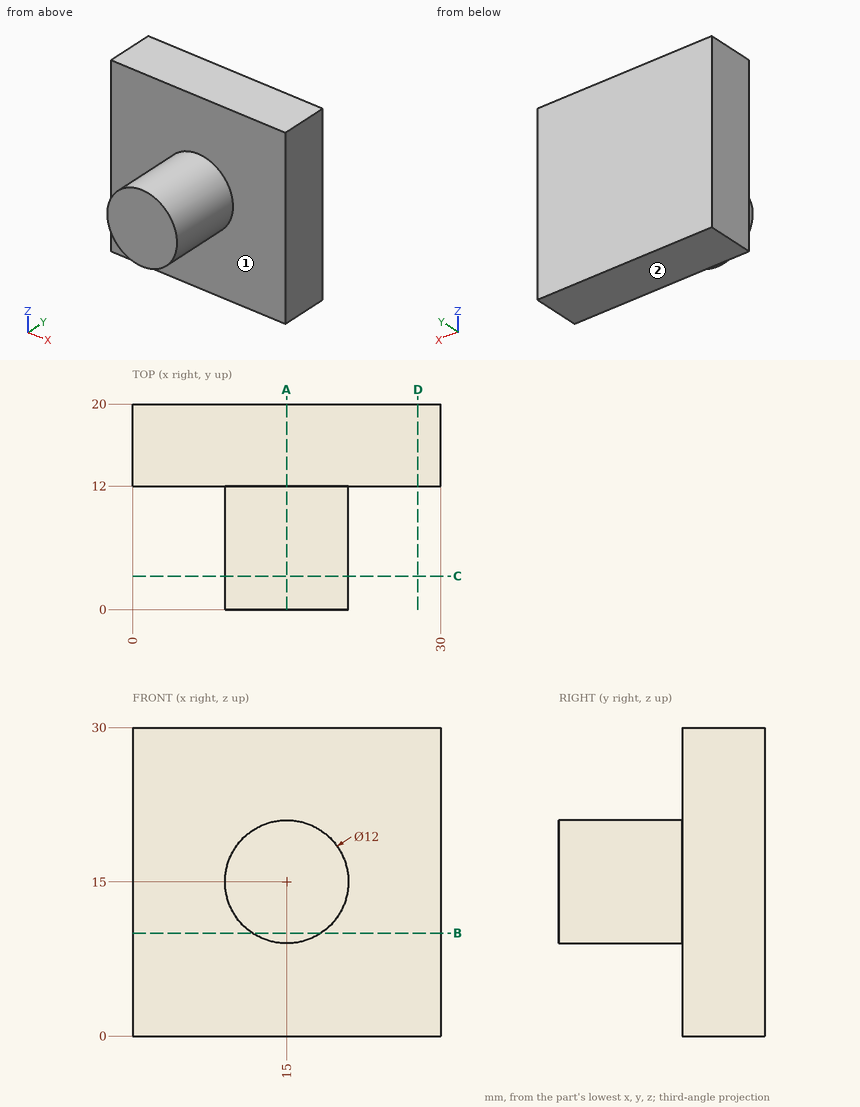
Geometry check sheet. Reference: drawing and pictorial views, mm from the part's lowest x, y, z. A direction names the side the tool comes from. Round coordinates to 2 decimals unless told otherwise and drop trailing zeros. Loops run counter-clockwise (first coordinate to the right, second up) from the corner with the lowest first, then second, coordinate; pieces in that order, holes last. Notation, with made-up numbers: M -28,55.25 L 4,55.25 A18 ccw 4,78.25 Z; hole C 20.25,83 d1. An arc over 180 degrees is marked long. Return JSON: item names as keys, results as strings. Group by question number.
(1) Section check D-D, the plane x = 27.75. Enter the section's corners in (y, z).
(2) Section check A-A, the plane x = 15. Enter the section's corners in (y, z), and give its area (3 significant figures).
(3) Section check B-B, the plane z = 10. Enter the section's corners in (x, y).
(4) Scan lines: line 1 along Y through (x, z) = (18.75, 28); line 2 along Z through (x, y) = (16.5, 8.75); line 3 along Z through (x, y) = (11.25, 2.25). Record each from-to range of solid material in increasing order. Write a range as [from, to].
(5) Set-up check for the marked faces 1 and 2: record each of +Z, -Z, +X, -X, +Y, -Y from which the full face is reachable in a straight line by a thin tool's end or side.
(6) Section check C-C, the plane y = 3.25. Enter the section's corners in (x, z), and give its area (3 significant figures).
(7) Go/stop test with flat-tipped pins: pin 1 (10 mm diameter, centred on x = 9.5, y = 2, fed in from +Z); pin 2 (10 mm diameter, centred on y = 3, z = 15, fed in from -X). Record where each tip stops, or that it passes through.
Data:
{
 "1": {"outline": "M 12,0 L 20,0 L 20,30 L 12,30 Z"},
 "2": {"outline": "M 0,9 L 12,9 L 12,0 L 20,0 L 20,30 L 12,30 L 12,21 L 0,21 Z", "area": "384 mm²"},
 "3": {"outline": "M 0,12 L 11.68,12 L 11.68,0 L 18.32,0 L 18.32,12 L 30,12 L 30,20 L 0,20 Z"},
 "4": {"line 1": "[12, 20]", "line 2": "[9.19, 20.81]", "line 3": "[10.32, 19.68]"},
 "5": {"face 1": "-Y", "face 2": "-Z, +X, -X, +Y, -Y"},
 "6": {"outline": "C 15,15 d12", "area": "113 mm²"},
 "7": {"pin 1": "z = 20.98", "pin 2": "x = 9"}
}
